Read the model definition and answer for the solid it produces. Units are mm, in the model's axes. Coordinates: 2 decimals unless noted, no trailing zeros. Order: outer loops, then holes, each group sorted by start corner. A loop starts at its lowest first (then second) coordinate and runs counter-clockwise, first axis right, second up. Notation, with made-up numbers: (38.5, -5.75) -> (74.5, -5.75) arc R17 ccw to (74.5, 10.25) -> close; hole circle Ø6 at (48.5, 81.5). An arc over 180 degrees is marked (long way). Answer in a Markdown table with one row per item.
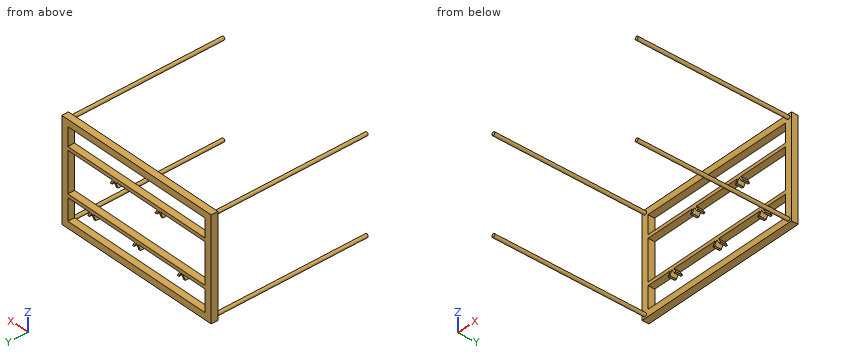
from build123d import *

# Parameters (mm, degrees)
SKETCH2_W           = 500
SKETCH2_H           = 300
BOSS_EXTRUDE1_DEPTH = 20
SKETCH5_R           = 5
BOSS_EXTRUDE2_DEPTH = 450
SKETCH7_W           = 460
SKETCH7_H           = 260
CUT_EXTRUDE1_DEPTH  = 20
SKETCH8_W           = 500
SKETCH8_H           = 10
BOSS_EXTRUDE3_DEPTH = 20
BOSS_EXTRUDE8_DEPTH = 20
BOSS_EXTRUDE9_DEPTH = 20
CUT_EXTRUDE6_DEPTH  = 20


with BuildPart() as part:
    # Sketch2 → Boss-Extrude1 (new body)
    with BuildSketch(Plane(origin=(0, 0, 0), x_dir=(1, 0, 0), z_dir=(0, 1, 0))):
        Rectangle(SKETCH2_W, SKETCH2_H)
    extrude(amount=BOSS_EXTRUDE1_DEPTH)

    # Sketch5 → Boss-Extrude2 (add)
    with BuildSketch(Plane(origin=(0, 0, 0), x_dir=(1, 0, 0), z_dir=(0, 1, 0))):
        with Locations((-240, 140)):
            Circle(SKETCH5_R)
        with Locations((240, 140)):
            Circle(SKETCH5_R)
        with Locations((-240, -140)):
            Circle(SKETCH5_R)
        with Locations((240, -140)):
            Circle(SKETCH5_R)
    extrude(amount=-BOSS_EXTRUDE2_DEPTH)

    # Sketch7 → Cut-Extrude1 (cut)
    with BuildSketch(Plane(origin=(0, 0, 0), x_dir=(-1, 0, 0), z_dir=(0, -1, 0))):
        Rectangle(SKETCH7_W, SKETCH7_H)
    extrude(amount=-CUT_EXTRUDE1_DEPTH, mode=Mode.SUBTRACT)

    # Sketch8 → Boss-Extrude3 (add)
    with BuildSketch(Plane(origin=(0, 0, 0), x_dir=(1, 0, 0), z_dir=(0, 1, 0))):
        with Locations((0, 60)):
            Rectangle(SKETCH8_W, SKETCH8_H)
        with Locations((0, -70)):
            Rectangle(SKETCH8_W, SKETCH8_H)
    extrude(amount=BOSS_EXTRUDE3_DEPTH)

    # Sketch13 → Boss-Extrude8 (add)
    with BuildSketch(Plane(origin=(0, 20, 0), x_dir=(1, 0, 0), z_dir=(0, 1, 0))):
        Polygon((75, -74.929562993), (87.929380819, -52.535218504), (62.070619181, -52.535218504), align=None)
        Polygon((-75, -74.929562993), (-62.070619181, -52.535218504), (-87.929380819, -52.535218504), align=None)
    extrude(amount=-BOSS_EXTRUDE8_DEPTH)

    # Sketch9 → Boss-Extrude9 (add)
    with BuildSketch(Plane(origin=(0, 0, 0), x_dir=(1, 0, 0), z_dir=(0, 1, 0))):
        Polygon((-150, 55), (-136.882070442, 77.720920485), (-163.117929558, 77.720920485), align=None)
        Polygon((13.117929558, 77.720920485), (-13.117929558, 77.720920485), (0, 55), align=None)
        Polygon((163.117929558, 77.720920485), (136.882070442, 77.720920485), (150, 55), align=None)
    extrude(amount=BOSS_EXTRUDE9_DEPTH)

    # Sketch14 → Cut-Extrude6 (cut)
    with BuildSketch(Plane(origin=(0, 0, 0), x_dir=(1, 0, 0), z_dir=(0, 1, 0))):
        Polygon((-150, 65), (-138.983359701, 84.081380727), (-161.016640299, 84.081380727), align=None)
        Polygon((0, 65), (11.016640299, 84.081380727), (-11.016640299, 84.081380727), align=None)
        Polygon((150, 65), (161.016640299, 84.081380727), (138.983359701, 84.081380727), align=None)
        Polygon((75, -65), (85.794817429, -46.302827755), (64.205182571, -46.302827755), align=None)
        Polygon((-75, -65), (-64.205182571, -46.302827755), (-85.794817429, -46.302827755), align=None)
    extrude(amount=CUT_EXTRUDE6_DEPTH, mode=Mode.SUBTRACT)


solid = part.part
Q1. The part is cut by section C-C (y = -324). Write down the section's boundary in (x, z), then the cut area to 3 significant figures.
Outcome:
| item | result |
|---|---|
| outline | circle Ø10 at (-240, -140); circle Ø10 at (-240, 140); circle Ø10 at (240, -140); circle Ø10 at (240, 140) |
| area | 314 mm² |
Q2. Consider line 1 (Y direction, x = 1, z = 130.5). Determine where the line is inside the solid, lowest interval first.
Outcome:
| item | result |
|---|---|
| line 1 | 0 to 20 |
Q3. The part is cut by section A-A (x = -40.5). Write down the section's boundary in (y, z), then the cut area to 3 significant figures.
Outcome:
| item | result |
|---|---|
| outline | (0, -150) -> (20, -150) -> (20, -130) -> (0, -130) -> close; (0, -65) -> (20, -65) -> (20, -55) -> (0, -55) -> close; (0, 65) -> (20, 65) -> (20, 75) -> (0, 75) -> close; (0, 130) -> (20, 130) -> (20, 150) -> (0, 150) -> close |
| area | 1,200 mm² |
Q4. Given pin 1 (10 mm diameter, centred on x = 102.5, z = 57, fed in from -Y), flat-ended and moving along its own axis, determine where the tip first touches the part or whether it passes through.
Outcome:
| item | result |
|---|---|
| pin 1 | through |
Q5. The part is cut by section B-B (z = -112). Write down the section's boundary in (x, y).
Outcome:
| item | result |
|---|---|
| outline | (-250, 0) -> (-230, 0) -> (-230, 20) -> (-250, 20) -> close; (230, 0) -> (250, 0) -> (250, 20) -> (230, 20) -> close |
